from build123d import *

# Parameters (mm, degrees)
F0_W     = 130
F0_H     = 90
F1_DEPTH = 20
F2_W     = 20
F2_H     = 90
F3_DEPTH = 10
F4_R     = 25.06944
F5_DEPTH = 20.001
F6_R     = 5.5
F7_DEPTH = 130.001
F9_DEPTH = 90.001


with BuildPart() as f1:
    # F0 (on Top) → F1 (new body)
    with BuildSketch(Plane.XY):
        Rectangle(F0_W, F0_H)
    extrude(amount=F1_DEPTH)

    # F2 (on face) → F3 (cut)
    with BuildSketch(Plane.XY.offset(20)):
        with Locations((-42.149333, 0)):
            Rectangle(F2_W, F2_H)
    extrude(amount=-F3_DEPTH, mode=Mode.SUBTRACT)

    # F4 (on face) → F5 (cut, through all)
    with BuildSketch(Plane.XY.offset(20)):
        Circle(F4_R)
    extrude(amount=-F5_DEPTH, mode=Mode.SUBTRACT)

    # F6 (on face) → F7 (cut, through all)
    with BuildSketch(Plane.YZ.offset(65)):
        with Locations((0, 10)):
            Circle(F6_R)
    extrude(amount=-F7_DEPTH, mode=Mode.SUBTRACT)

    # F8 (on face) → F9 (cut, through all)
    with BuildSketch(Plane.XZ.offset(45)):
        Polygon((47.662321, 20), (41.323712, 20), (35.550209, 10), (53.435824, 10), align=None)
    extrude(amount=-F9_DEPTH, mode=Mode.SUBTRACT)


solid = f1.part
Verification items for the finished model (mm, model axes). A direction names the side the tool comes from. Coordinates: 2 decimals unless noted, no trailing zeros. Order: outer loops, then holes, each group sorted by start corner. A loop starts at its lowest first (then second) coordinate and runs counter-clockwise, first axis right, second up. Notation, with made-up numbers: M 48.5,16.5 L 53.5,16.5 A22 ccw 53.5,36.5 Z; hole C 31,28.25 d2. An arc over 180 degrees is marked long. Return JSON: item names as keys, results as strings.
1) Cross-section at C-C, the plane x = 28.5. Record the boundary of the cut face in (y, z).
Answer list:
{"outline": "M -45,0 L 45,0 L 45,20 L -45,20 Z; hole C 0,10 d11"}
2) Release check for a two-part mould opening along X. For faces 1 (the flat face through (-42, -25, 10)), 2 (the flat face through (-1, 45, 10)), 3 (the flat face through (-65, -1, 3)), 4 (the flat face through (44, 25, 10)) record: +X half, -X half, draft (parallel to the pull), parting line (faces both ways), or undercut.
Answer list:
{"face 1": "undercut", "face 2": "draft", "face 3": "-X half", "face 4": "undercut"}
3) Gauge pin test, flat ends, axial feed: pin 1 (10 mm diameter, centred on x = -43, y = -7.5, fed in from +Z); pin 2 (16 mm diameter, centred on x = -39, y = -16.5, fed in from +Z); pin 3 (9 mm diameter, centred on y = 0, z = 10, fed in from +X). Record the tip position at first contact, or that the pin passes through.
Answer list:
{"pin 1": "z = 10", "pin 2": "z = 20", "pin 3": "through"}
4) Cross-section at D-D, the plane y = 20. Record the boundary of the cut face in (x, z).
Answer list:
{"outline": "M -65,0 L -15.12,0 L -15.12,20 L -32.15,20 L -32.15,10 L -52.15,10 L -52.15,20 L -65,20 Z; M 15.12,0 L 65,0 L 65,20 L 47.66,20 L 53.44,10 L 35.55,10 L 41.32,20 L 15.12,20 Z"}
5) Cross-section at A-A, the plane x = 0. Record the boundary of the cut face in (y, z), and give its area (3 significant figures).
Answer list:
{"outline": "M -45,0 L -25.07,0 L -25.07,20 L -45,20 Z; M 25.07,0 L 45,0 L 45,20 L 25.07,20 Z", "area": "797 mm2"}
6) Cross-section at B-B, the plane y = 0. Record the boundary of the cut face in (x, z), and give its area (3 significant figures).
Answer list:
{"outline": "M -65,0 L -25.07,0 L -25.07,4.5 L -65,4.5 Z; M -65,15.5 L -52.15,15.5 L -52.15,20 L -65,20 Z; M -32.15,15.5 L -25.07,15.5 L -25.07,20 L -32.15,20 Z; M 25.07,0 L 65,0 L 65,4.5 L 25.07,4.5 Z; M 25.07,15.5 L 38.73,15.5 L 41.32,20 L 25.07,20 Z; M 47.66,20 L 50.26,15.5 L 65,15.5 L 65,20 Z", "area": "589 mm2"}
7) Thickness scan on L1, parallel to X at y = 1, z = 4; L2, parallel to Z at x = 58, y = -0.5; L3, parallel to X at y = 35, z = 10.5. Record the ranges inside material, lowest first. Write a range as [from, to].
Answer list:
{"L1": "[-65, -25.05], [25.05, 65]", "L2": "[0, 4.52], [15.48, 20]", "L3": "[-65, -52.15], [-32.15, 35.84], [53.15, 65]"}
8) Access from +Z, -Z, +X, -X, +Y, -Y to the whole of each face (thin tool, end or side, straight path). Record for faces 5 (the flat face through (-59, 1, 20)), 6 (the flat face through (44, -26, 10)), 7 (the flat face through (-52.149, -1, 16)).
Answer list:
{"face 5": "+Z, +X, -X, +Y, -Y", "face 6": "+Y, -Y", "face 7": "+Z, +Y, -Y"}
